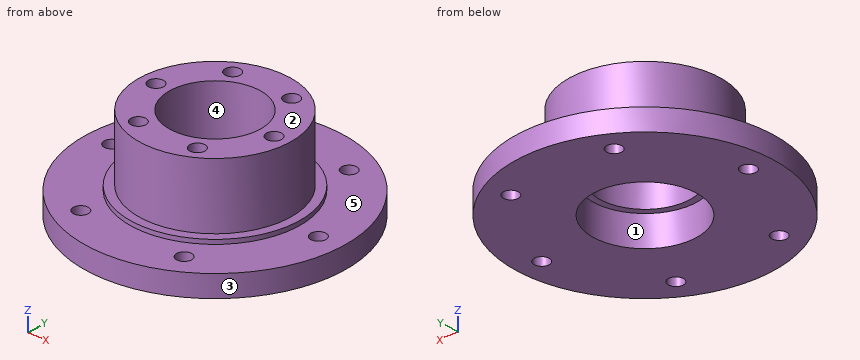
from build123d import *

# Parameters (mm, degrees)
SKETCH1_R           = 30
BOSS_EXTRUDE1_DEPTH = 5
SKETCH2_R           = 19.5
BOSS_EXTRUDE2_DEPTH = 1
SKETCH3_R           = 17.5
BOSS_EXTRUDE3_DEPTH = 15
SKETCH4_R           = 12.025
CUT_EXTRUDE1_DEPTH  = 7
SKETCH5_R           = 10.5
CUT_EXTRUDE2_DEPTH  = 45.676615807
SKETCH6_R           = 1.75
CUT_EXTRUDE3_DEPTH  = 46.343136195
SKETCH7_R           = 1.75
CUT_EXTRUDE4_DEPTH  = 12


with BuildPart() as part:
    # Sketch1 → Boss-Extrude1 (new body)
    with BuildSketch(Plane.XY):
        Circle(SKETCH1_R)
    extrude(amount=BOSS_EXTRUDE1_DEPTH)

    # Sketch2 → Boss-Extrude2 (add)
    with BuildSketch(Plane.XY.offset(5)):
        Circle(SKETCH2_R)
    extrude(amount=BOSS_EXTRUDE2_DEPTH)

    # Sketch3 → Boss-Extrude3 (add)
    with BuildSketch(Plane.XY.offset(6)):
        Circle(SKETCH3_R)
    extrude(amount=BOSS_EXTRUDE3_DEPTH)

    # Sketch4 → Cut-Extrude1 (cut)
    with BuildSketch(Plane(origin=(0, 0, 0), x_dir=(-1, 0, 0), z_dir=(0, 0, -1))):
        Circle(SKETCH4_R)
    extrude(amount=-CUT_EXTRUDE1_DEPTH, mode=Mode.SUBTRACT)

    # Sketch5 → Cut-Extrude2 (cut, through all)
    with BuildSketch(Plane(origin=(0, 0, 7), x_dir=(-1, 0, 0), z_dir=(0, 0, -1))):
        Circle(SKETCH5_R)
    extrude(amount=-CUT_EXTRUDE2_DEPTH, mode=Mode.SUBTRACT)

    # Sketch6 → Cut-Extrude3 (cut, through all)
    with BuildSketch(Plane.XY.offset(5)):
        with Locations((24.5, 0)):
            Circle(SKETCH6_R)
        with Locations((12.25, -21.217622393)):
            Circle(SKETCH6_R)
        with Locations((-12.25, -21.217622393)):
            Circle(SKETCH6_R)
        with Locations((-24.5, 0)):
            Circle(SKETCH6_R)
        with Locations((-12.25, 21.217622393)):
            Circle(SKETCH6_R)
        with Locations((12.25, 21.217622393)):
            Circle(SKETCH6_R)
    extrude(amount=-CUT_EXTRUDE3_DEPTH, mode=Mode.SUBTRACT)

    # Sketch7 → Cut-Extrude4 (cut)
    with BuildSketch(Plane.XY.offset(21)):
        with Locations((14, 0)):
            Circle(SKETCH7_R)
        with Locations((7, -12.124355653)):
            Circle(SKETCH7_R)
        with Locations((-7, -12.124355653)):
            Circle(SKETCH7_R)
        with Locations((-14, 0)):
            Circle(SKETCH7_R)
        with Locations((-7, 12.124355653)):
            Circle(SKETCH7_R)
        with Locations((7, 12.124355653)):
            Circle(SKETCH7_R)
    extrude(amount=-CUT_EXTRUDE4_DEPTH, mode=Mode.SUBTRACT)


solid = part.part
Geometry: final body of the model. Coordinates: model frame, mm. Face numbers are marked on the shaded views. A direction names the side the tool comes from. Give positions to 0.01 mm unless a question says otherwise; leave off trailing zeros. Write each loop counter-clockwise with the first axis right and the second up, starting at its lowest first coordinate (ties: lowest second). Pieces come first, ordered by that corner, then holes. Notation, with made-up numbers: (40, 37.5) - (93, 37.5) arc R23 cw to (93, 63.5) - close; hole circle Ø3 at (45.25, 4.25). An arc over 180 degrees is marked (long way). Return JSON: item names as keys, results as strings. Group by question number.
1) Section C-C on z = 17.5. Return the cut outline in (x, y), plus the area to 3 significant figures.
2) Line query: line 1 (X direction, y = -21.5, z = 1.5); line 2 (Z direction, x = 19, y = 21.5); line 3 (X direction, y = 11, z = 11). Output: solid intervals per line, ascending.
3) Section A-A on x = 0. Return the cut outline in (y, z) (3 decimals), plus the area to 3 significant figures.
4) Mould query, pull axis Y, two halves, no side actions, for the marked faces 1, 2 and 3. Classes: released by +Y, released by -Y, zero draft, split by the parting line, or undercut.
5) First-contact query: P1, Ø12, axis at x = 1, y = -4.5, coming from the -Z side; P2, Ø6, axis at x = -3.5, z = 7.5, coming from the -Y side; P3, Ø1, axis at x = 7.5, y = -11.5, coming from the +Z side; P4, Ø3, axis at x = 12.25, y = -21.22, coming from the -Z side. Flat tips, straight axial feed; report the tip coordinate or a pass-through.
6) Set-up query: the marked faces 4 and 5. Return all of +Z, -Z, +X, -X, +Y, -Y with unobstructed straight access to the full face (end or side cutting, diameter ignored); none if empty.
7) Section B-B on y = 8. Return the cut outline in (x, z), plus the area to 3 significant figures.
8) Section D-D on x = -8. Return the cut outline in (y, z).
Filled in:
{
 "1": {"outline": "circle Ø35 at (0, 0); hole circle Ø3.5 at (-14, 0); hole circle Ø21 at (0, 0); hole circle Ø3.5 at (-7, -12.12); hole circle Ø3.5 at (-7, 12.12); hole circle Ø3.5 at (7, -12.12); hole circle Ø3.5 at (7, 12.12); hole circle Ø3.5 at (14, 0)", "area": "558 mm^2"},
 "2": {"line 1": "x = -20.92 to -13.98, -10.52 to 10.52, 13.98 to 20.92", "line 2": "z = 0 to 5", "line 3": "x = -13.61 to -8.34, -5.66 to 5.66, 8.34 to 13.61"},
 "3": {"outline": "(-30, 0) - (-12.025, 0) - (-12.025, 7) - (-10.5, 7) - (-10.5, 21) - (-17.5, 21) - (-17.5, 6) - (-19.5, 6) - (-19.5, 5) - (-30, 5) - close; (10.5, 7) - (12.025, 7) - (12.025, 0) - (30, 0) - (30, 5) - (19.5, 5) - (19.5, 6) - (17.5, 6) - (17.5, 21) - (10.5, 21) - close", "area": "402 mm^2"},
 "4": {"face 1": "undercut", "face 2": "zero draft", "face 3": "split by the parting line"},
 "5": {"P1": "stops at z = 7", "P2": "stops at y = -29.94", "P3": "stops at z = 9", "P4": "passes through"},
 "6": {"face 4": "+Z, -Z", "face 5": "+Z"},
 "7": {"outline": "(-28.91, 0) - (-8.98, 0) - (-8.98, 7) - (-6.8, 7) - (-6.8, 21) - (-15.56, 21) - (-15.56, 6) - (-17.78, 6) - (-17.78, 5) - (-28.91, 5) - close; (6.8, 7) - (8.98, 7) - (8.98, 0) - (28.91, 0) - (28.91, 5) - (17.78, 5) - (17.78, 6) - (15.56, 6) - (15.56, 21) - (6.8, 21) - close", "area": "476 mm^2"},
 "8": {"outline": "(-28.91, 0) - (-8.98, 0) - (-8.98, 7) - (-6.8, 7) - (-6.8, 21) - (-10.69, 21) - (-10.69, 9) - (-13.56, 9) - (-13.56, 21) - (-15.56, 21) - (-15.56, 6) - (-17.78, 6) - (-17.78, 5) - (-28.91, 5) - close; (6.8, 7) - (8.98, 7) - (8.98, 0) - (28.91, 0) - (28.91, 5) - (17.78, 5) - (17.78, 6) - (15.56, 6) - (15.56, 21) - (13.56, 21) - (13.56, 9) - (10.69, 9) - (10.69, 21) - (6.8, 21) - close"}
}
